Build history of the part. All positions in model axes, mm. A direction names the side the tool comes from. Coordinates: 2 decimals unless noted, no trailing zeros. Loops run counter-clockwise (first coordinate to the right, second up) from the corner with the lowest first, then second, coordinate; pieces in that order, holes last.
(1) Slice it at C-C (z = 1.1). Give the number of separate pieces and of enclosed holes in the cut face, and give its area (3 significant figures).
(2) Wall check: L1, parallel to Y at x = 1, z = 3.2; L2, parallel to X at y = -11, z = 0.75; L3, parallel to Y at x = -10.5, z = 3.8. Give the ranges that are in metal, low to high.
(3) Slice it at D-D (x = 24.5). Give the cut face in (y, z), and give its area (3 significant figures).
(4) Tool access for faces 1 (the face through (0, 43.026, 2)), 2 (the face through (-19.125, 17, 2)): list every direction of +Z, -Z, +X, -X, +Y, -Y with a clear straight run to the whole face (end or side of a thin tool).
(5) Two-plate mould, pull along X, no slides. Class faces 3 (the face through (13.27, 9.75, 1.97)), 4 (the face through (-5.877, 17.39, 1.972)), 5 (the face through (6, 14, 4)), 6 (the face through (-26.625, 16, 2)): pulls with the +X half, pulls with the -X half, needs draft (parallel to the pull), parting line crosses it, or undercut.
(6) Slice it at A-A (y = 0). Give the cut face in (x, z), and give its area (3 significant figures).
(7) Flat gauge pins, fed straight in: P1, Ø2, axis at y = 23, z = 2, coming from the -X side; P2, Ø2, axis at x = -6, z = 3, coming from the -Y side; P3, Ø3, axis at x = 15, y = 2.5, coming from the -Z side; P4, Ø2, axis at y = 14, z = 1, coming from the +X side. Where does each tip first touch, or does it go through?
(8) Slice it at B-B (x = 12.5). Give the cut face in (y, z), and give its area (3 significant figures).
from build123d import *

# Parameters (mm, degrees)
SKETCH1_R           = 1.5
BOSS_EXTRUDE1_DEPTH = 4


with BuildPart() as part:
    # Sketch1 → Boss-Extrude1 (new body)
    with BuildSketch(Plane.XY):
        with BuildLine():
            ThreePointArc((-26.624535685, -6.97381528), (-29.02618472, -13.624535685), (-22.375464315, -16.02618472))
            Line((-22.375464315, -16.02618472), (-22.205082013, -15.942223704))
            Line((-22.205082013, -15.942223704), (-4.420251148, -7.178212035))
            ThreePointArc((-4.420251148, -7.178212035), (0, -6.148238779), (4.420251148, -7.178212035))
            Line((4.420251148, -7.178212035), (22.205082013, -15.942223704))
            Line((22.205082013, -15.942223704), (22.375464315, -16.02618472))
            ThreePointArc((22.375464315, -16.02618472), (29.02618472, -13.624535685), (26.624535685, -6.97381528))
            Line((26.624535685, -6.97381528), (26.624535685, 38.02618472))
            ThreePointArc((26.624535685, 38.02618472), (25.160069591, 41.561718626), (21.624535685, 43.02618472))
            Line((21.624535685, 43.02618472), (-21.624535685, 43.02618472))
            ThreePointArc((-21.624535685, 43.02618472), (-25.160069591, 41.561718626), (-26.624535685, 38.02618472))
            Line((-26.624535685, 38.02618472), (-26.624535685, -6.97381528))
        make_face()
        with Locations((-24.5, -11.5)):
            Circle(SKETCH1_R, mode=Mode.SUBTRACT)
        with Locations((24.5, -11.5)):
            Circle(SKETCH1_R, mode=Mode.SUBTRACT)
        Circle(SKETCH1_R, mode=Mode.SUBTRACT)
        with BuildLine():
            Line((14.374535685, -1.22381528), (2.124535685, 4.52618472))
            ThreePointArc((2.124535685, 4.52618472), (0, 5), (-2.124535685, 4.52618472))
            Line((-2.124535685, 4.52618472), (-14.374535685, -1.22381528))
            Line((-14.374535685, -1.22381528), (-2.097868645, 10.785812849))
            ThreePointArc((-2.097868645, 10.785812849), (0, 11.641297251), (2.097868645, 10.785812849))
            Line((2.097868645, 10.785812849), (14.374535685, -1.22381528))
        make_face(mode=Mode.SUBTRACT)
        with BuildLine():
            Line((-6.73171968, 15.226590291), (-19.124535685, 2.558215038))
            Line((-19.124535685, 2.558215038), (-19.124535685, 31.546592884))
            Line((-19.124535685, 31.546592884), (-6.778366633, 19.468974534))
            ThreePointArc((-6.778366633, 19.468974534), (-5.876416612, 17.357443313), (-6.73171968, 15.226590291))
        make_face(mode=Mode.SUBTRACT)
        with BuildLine():
            Line((19.124535685, 31.546592884), (19.124535685, 4.020746784))
            Line((19.124535685, 4.020746784), (7.24778827, 15.639154236))
            ThreePointArc((7.24778827, 15.639154236), (6.345656915, 17.783669834), (7.24778827, 19.928185432))
            Line((7.24778827, 19.928185432), (19.124535685, 31.546592884))
        make_face(mode=Mode.SUBTRACT)
        with BuildLine():
            Line((-1.833941699, 24.523340745), (-14.124535685, 36.546592884))
            Line((-14.124535685, 36.546592884), (14.124535685, 36.546592884))
            Line((14.124535685, 36.546592884), (2.408442543, 24.569987698))
            ThreePointArc((2.408442543, 24.569987698), (0.296911322, 23.668037677), (-1.833941699, 24.523340745))
        make_face(mode=Mode.SUBTRACT)
    extrude(amount=BOSS_EXTRUDE1_DEPTH)


solid = part.part
Response values:
1. separate pieces: 1
1. enclosed holes: 7
1. area: 2,210 mm2
2. L1: y = -6.2 to -1.12, 1.12 to 4.9, 11.47 to 23.76, 36.55 to 43.03
2. L2: x = -29.47 to -25.91, -23.09 to -12.18, 12.18 to 23.09, 25.91 to 29.47
2. L3: y = -10.17 to 0.59, 2.57 to 11.37, 23.11 to 33, 36.55 to 43.03
3. outline: (-16.5, 0) - (-13, 0) - (-13, 4) - (-16.5, 4) - close; (-10, 0) - (42.12, 0) - (42.12, 4) - (-10, 4) - close
3. area: 222 mm2
4. face 1: +Z, -Z, +X, -X, +Y
4. face 2: +Z, -Z
5. face 3: undercut
5. face 4: undercut
5. face 5: needs draft
5. face 6: pulls with the -X half
6. outline: (-26.62, 0) - (-13.12, 0) - (-13.12, 4) - (-26.62, 4) - close; (-11.77, 0) - (-1.5, 0) - (-1.5, 4) - (-11.77, 4) - close; (1.5, 0) - (11.77, 0) - (11.77, 4) - (1.5, 4) - close; (13.12, 0) - (26.62, 0) - (26.62, 4) - (13.12, 4) - close
6. area: 190 mm2
7. P1: stops at x = -26.62
7. P2: stops at y = -8.45
7. P3: stops at z = 0
7. P4: stops at x = 26.62
8. outline: (-11.16, 0) - (-0.34, 0) - (-0.34, 4) - (-11.16, 4) - close; (0.61, 0) - (10.5, 0) - (10.5, 4) - (0.61, 4) - close; (25.07, 0) - (34.89, 0) - (34.89, 4) - (25.07, 4) - close; (36.55, 0) - (43.03, 0) - (43.03, 4) - (36.55, 4) - close
8. area: 148 mm2
